Geometry: final body of the model. Coordinates: model frame, mm. Face numbers are marked on the shaded views. A direction names the side the tool comes from. Coordinates: 2 decimals unless noted, no trailing zeros. Order: outer loops, then holes, each group sorted by start corner. A loop starts at its lowest first (then second) coordinate and runs counter-clockwise, first axis right, second up. Notation, with made-up numbers: M 0.5,4 L 7.5,4 A26 ccw 7.5,24 Z; hole C 71,-15 d3. An arc over 180 degrees is marked long. Use CSV: the item, a comma, the result in double quotes. Start each with the question number.
1. Section query C-C on y = -23.5. Return the cut outline in (x, z).
2. Section query B-B on y = -5.5. Return the cut outline in (x, z).
3. Pull-direction query (Y, two-part tool) for the marked faces 3, 4, 5 and 6; classes: pulls with the +Y half, pulls with the -Y half, needs draft (parallel to the pull), parting line crosses it, or undercut.
4. Material intervals for line 1 (X direction, y = -10.5, z = 3.5); line 2 (Y direction, x = -5, z = 1.5); line 3 (X direction, y = -10, z = 1.5), sorted ascending.
5. Set-up query: the marked faces 1 and 2. Return all of +Z, -Z, +X, -X, +Y, -Y with unobstructed straight access to the full face (end or side cutting, diameter ignored); none if empty.
6. Section query A-A on x = -8. Return the cut outline in (y, z).
7. First-contact query: P1, Ø1.5, axis at x = 0, z = 3, coming from the -Y side; P2, Ø3, axis at x = 9, z = 1, coming from the +Y side. Flat tips, straight axial feed; report the tip coordinate or a pass-through.
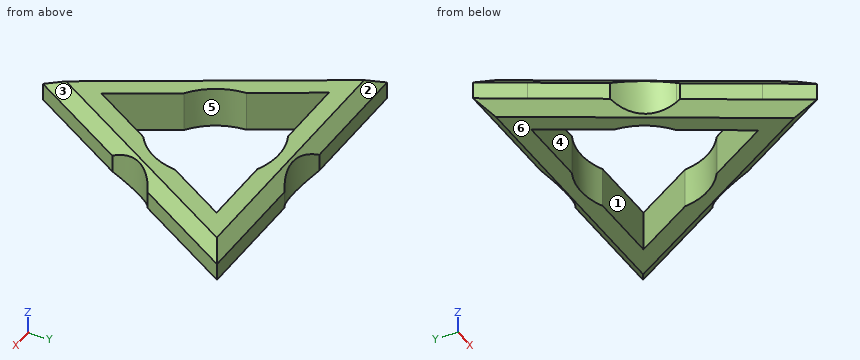
from build123d import *

# Parameters (mm, degrees)
F1_DEPTH = 7
F2_SIZE  = 2


with BuildPart() as f1:
    # F0 (on Top) → F1 (new body)
    with BuildSketch(Plane.XY):
        with BuildLine():
            Line((-5.2907653123, 15.0261512026), (-17.7863569535, 15.0261512026))
            Line((-17.7863569535, 15.0261512026), (-21.9062071393, 7.8903613612))
            Line((-21.9062071393, 7.8903613612), (-15.6584113187, -2.9311384354))
            ThreePointArc((-15.6584113187, -2.9311384354), (-11.782946139, -6.4350487366), (-10.3462820464, -11.4582562819))
            ThreePointArc((-10.3462820464, -11.4582562819), (-10.3516245386, -11.7768136709), (-10.3676460064, -12.0950127672))
            Line((-10.3676460064, -12.0950127672), (-4.1198501858, -22.9165125638))
            Line((-4.1198501858, -22.9165125638), (4.1198501858, -22.9165125638))
            Line((4.1198501858, -22.9165125638), (10.3680051395, -12.0943907304))
            ThreePointArc((10.3680051395, -12.0943907304), (11.6193871206, -6.7084562819), (15.6580521856, -2.9317604722))
            Line((15.6580521856, -2.9317604722), (21.9062071393, 7.8903613612))
            Line((21.9062071393, 7.8903613612), (17.7863569535, 15.0261512026))
            Line((17.7863569535, 15.0261512026), (5.2907653123, 15.0261512026))
            ThreePointArc((5.2907653123, 15.0261512026), (0, 13.4165125638), (-5.2907653123, 15.0261512026))
        make_face()
        with BuildLine():
            ThreePointArc((-4.7301378537, 9.9310521036), (0, 11), (4.7301378537, 9.9310521036))
            Line((4.7301378537, 9.9310521036), (17.2010868161, 9.9310521036))
            Line((17.2010868161, 9.9310521036), (10.9656123349, -0.8691065071))
            ThreePointArc((10.9656123349, -0.8691065071), (9.5262794416, -5.5), (6.2354744812, -9.0619455965))
            Line((6.2354744812, -9.0619455965), (0, -19.8621042073))
            Line((0, -19.8621042073), (-6.2354744812, -9.0619455965))
            ThreePointArc((-6.2354744812, -9.0619455965), (-9.5262794416, -5.5), (-10.9656123349, -0.8691065071))
            Line((-10.9656123349, -0.8691065071), (-17.2010868161, 9.9310521036))
            Line((-17.2010868161, 9.9310521036), (-4.7301378537, 9.9310521036))
        make_face(mode=Mode.SUBTRACT)
        Polygon((-17.7863569535, 15.0261512026), (-26.0260573251, 15.0261512026), (-21.9062071393, 7.8903613612), align=None)
        Polygon((26.0260573251, 15.0261512026), (17.7863569535, 15.0261512026), (21.9062071393, 7.8903613612), align=None)
        Polygon((4.1198501858, -22.9165125638), (-4.1198501858, -22.9165125638), (0, -30.0523024052), align=None)
    extrude(amount=F1_DEPTH)

    # F2 (call 1 of 5: OpenCascade refuses the feature's edges together)
    f2_edges = [f1.edges().sort_by_distance(p)[0] for p in [
        (-20.842234, 6.047506, 7),
        (-15.658411, 15.026151, 7),
    ]]
    chamfer(f2_edges, length=F2_SIZE)

    # F2#2 (call 2 of 5)
    f2_2_edges = [f1.edges().sort_by_distance(p)[0] for p in [
        (-5.183823, -21.073658, 0),
    ]]
    chamfer(f2_2_edges, length=F2_SIZE)

    # F2#3 (call 3 of 5)
    f2_3_edges = [f1.edges().sort_by_distance(p)[0] for p in [
        (-15.658411, 15.026151, 0),
    ]]
    chamfer(f2_3_edges, length=F2_SIZE)

    # F2#4 (call 4 of 5)
    f2_4_edges = [f1.edges().sort_by_distance(p)[0] for p in [
        (20.842055, 6.047195, 7),
    ]]
    chamfer(f2_4_edges, length=F2_SIZE)

    # F2#5 (call 5 of 5)
    f2_5_edges = [f1.edges().sort_by_distance(p)[0] for p in [
        (20.842055, 6.047195, 0),
    ]]
    chamfer(f2_5_edges, length=F2_SIZE)


solid = f1.part
Results list:
1,outline,"M -3.78,2 L -1.47,0 L 1.47,0 L 3.78,2 L 3.78,5 L 1.47,7 L -1.47,7 L -3.78,5 Z"
2,outline,"M -12.45,0.5 L -11.87,0 L -9.53,0 L -9.53,7 L -11.87,7 L -12.45,6.5 Z; M 9.53,0 L 11.87,0 L 12.45,0.5 L 12.45,6.5 L 11.87,7 L 9.53,7 Z"
3,face 3,"pulls with the -Y half"
3,face 4,"undercut"
3,face 5,"undercut"
3,face 6,"needs draft"
4,line 1,"x = -10.39 to -5.41, 5.41 to 10.4"
4,line 2,"y = -20.39 to -11.2, 9.93 to 14.53"
4,line 3,"x = -10.46 to -5.69, 5.69 to 10.46"
5,face 1,"+Z, -Z"
5,face 2,"+Z, +X, -X, +Y"
6,outline,"M -16.2,2 L -12.2,0 L -7.55,0 L -7.55,7 L -12.2,7 L -16.2,5 Z; M 9.93,0 L 13.03,0 L 15.03,2 L 15.03,5 L 13.03,7 L 9.93,7 Z"
7,P1,"stops at y = -30.05"
7,P2,"stops at y = 15.03"
